from build123d import *

# Parameters (mm, degrees)
F1_DEPTH       = 25.4
F3_D           = 7.62
F6_D           = 4.445
F6_CSINK_D     = 8.382
F6_CSINK_ANGLE = 90
F7_D           = 4.445
F7_CSINK_D     = 8.382
F7_CSINK_ANGLE = 90


with BuildPart() as f1:
    # F0 (on Top) → F1 (new body)
    with BuildSketch(Plane.XY):
        Polygon((-10.795, 24.13), (-41.275, 24.13), (-41.275, 19.05), (-15.875, 19.05), (-15.875, 0), (15.875, 0), (15.875, 19.05), (41.275, 19.05), (41.275, 24.13), (10.795, 24.13), (10.795, 2.54), (-10.795, 2.54), align=None)
    extrude(amount=F1_DEPTH)

    # F3 (through all)
    with Locations(Plane.XZ):
        with Locations((0, 12.7)):
            Hole(F3_D / 2)

    # F6 (through all)
    with Locations(Plane.XZ.offset(-19.05)):
        with Locations((-28.575, 12.7)):
            CounterSinkHole(F6_D / 2, F6_CSINK_D / 2, counter_sink_angle=F6_CSINK_ANGLE)

    # F7 (through all)
    with Locations(Plane.XZ.offset(-19.05)):
        with Locations((28.575, 12.7)):
            CounterSinkHole(F7_D / 2, F7_CSINK_D / 2, counter_sink_angle=F7_CSINK_ANGLE)


solid = f1.part
The listing builds one solid part. Answer for the finished solid, in the listing's coordinates (mm). A direction names the side the tool comes from. Give positions to 0.01 mm unless a question says otherwise; leave off trailing zeros. Write each loop counter-clockwise with the first axis right and the second up, starting at its lowest first coordinate (ties: lowest second). Pieces come first, ordered by that corner, then holes.
1) A tool of negligible diameter and unlimited length cuts with its end or side. For faces 4 (the face through (10.795, 13, 13)), 5 (the face through (23, 19.05, 13)), 6 (the face through (-32, 19.05, 10)), from which of +Z, -Z, +X, -X, +Y, -Y can it reach the whole face along a straight path? Write none if from no direction.
2) Given P1, Ø12.5, axis at x = -32, z = 10, coming from the -Y side; P2, Ø1.5, axis at y = 15.5, z = 7, coming from the -X side (3 decimals); P3, Ø5, axis at x = 28.575, z = 12.7, coming from the -Y side; P4, Ø6, axis at x = 0, z = 12.7, coming from the +Y side, each flat-ended and moving along its own axis, determine where each tip first touches the part or whether it passes through.
3) Section C-C (z = 18.25) is taken. Write down the section's boundary in (x, y) (3 decimals), and give its area (3 significant figures).
4) Find the intervals of material crossed by L1, parallel to X at y = 22.7, z = 12.7 (1 decimal); L2, parallel to X at y = 17.5, z = 21.5 (3 decimals); L3, parallel to X at y = 21.5, z = 15.5 (3 decimals), in increasing order.
5) Section B-B (x = 0) is taken. Write down the section's boundary in (y, z), and give its area (3 significant figures).
6) For a pull along X with two mould halves and no side action, classify faces 1 (the face through (-41.275, 22, 13)), 2 (the face through (41.275, 22, 13)), 3 (the face through (26.455, 22.596, 13.368)) as pulls with the +X half, pulls with the -X half, needs draft (parallel to the pull), parting line crosses it, or undercut.
7) Section A-A (z = 12.7) is taken. Count the separate pieces of the cut face and the enclosed holes in it, and give its area (3 significant figures).
8) Section D-D (x = -18) is taken. Write down the section's boundary in (y, z), and give its area (3 significant figures).
Response:
1. face 4: +Z, -Z, +Y
1. face 5: +Z, -Z, +X, -Y
1. face 6: +Z, -Z, -X, -Y
2. P1: stops at y = 19.05
2. P2: stops at x = -15.875
2. P3: stops at y = 20.74
2. P4: passes through
3. outline: (-41.275, 19.05) - (-15.875, 19.05) - (-15.875, 0) - (15.875, 0) - (15.875, 19.05) - (41.275, 19.05) - (41.275, 24.13) - (10.795, 24.13) - (10.795, 2.54) - (-10.795, 2.54) - (-10.795, 24.13) - (-41.275, 24.13) - close
3. area: 558 mm2
4. L1: x = -41.3 to -30.8, -26.4 to -10.8, 10.8 to 26.4, 30.8 to 41.3
4. L2: x = -15.875 to -10.795, 10.795 to 15.875
4. L3: x = -41.275 to -10.795, 10.795 to 41.275
5. outline: (0, 0) - (2.54, 0) - (2.54, 8.89) - (0, 8.89) - close; (0, 16.51) - (2.54, 16.51) - (2.54, 25.4) - (0, 25.4) - close
5. area: 45.2 mm2
6. face 1: pulls with the -X half
6. face 2: pulls with the +X half
6. face 3: undercut
7. separate pieces: 4
7. enclosed holes: 0
7. area: 486 mm2
8. outline: (19.05, 0) - (24.13, 0) - (24.13, 25.4) - (19.05, 25.4) - close
8. area: 129 mm2
